The listing builds one solid part. Answer for the finished solid, in the listing's coordinates (mm). Face numbers are marked on the shaded views. Round coordinates to 2 decimals unless told otherwise and drop trailing zeros. Use a Markdown table: item, result. Add a question column.
Q1. Consider line 1 (Y direction, x = 0, z = 1.75) (1 decimal); line 2 (X direction, y = 39, z = 5.25); line 3 (Y direction, x = 20, z = 0.5). Determine where each line is inside the solid, lowest interval first.
Q2. Given pin 1 Ø5 at (y, z) = (62, 7.5) entering from +X; pin 2 Ø5 at (x, y) = (0, 133.35) entering from +Z; pin 3 Ø15 at (x, y) = (0.5, 5.5) entering from +Z, each flat-ended and moving along its own axis, determine where each tip first touches the part or whether it passes through.
Q3. For a pull along Z with two mould halves and no side action, classify the marked faces 1 and 2 as released by +Z, released by -Z, zero draft, split by the parting line, or undercut.
Q4. Section A-A on x = 48 is taken. Give the number of separate pieces and of enclosed holes in the cut face, then the cut area to 3 significant figures.
from build123d import *

# Parameters (mm, degrees)
SKETCH1_R           = 1.5875
BOSS_EXTRUDE1_DEPTH = 6.35
BOSS_EXTRUDE2_DEPTH = 133.35
CUT_EXTRUDE1_DEPTH  = 133.35
SKETCH5_RX          = 30.163516005
SKETCH5_RY          = 6.87067886
CUT_EXTRUDE2_DEPTH  = 216.619671093
BOSS_EXTRUDE3_DEPTH = 3.175
CUT_EXTRUDE3_START  = -7.9375
CUT_EXTRUDE3_DEPTH  = 7.9375
FILLET1_R           = 3.175


with BuildPart() as part:
    # Sketch1 → Boss-Extrude1 (new body)
    with BuildSketch(Plane.XY):
        with BuildLine():
            Line((150.084701559, -26.463982276), (6.230674922, -1.098636097))
            ThreePointArc((6.230674922, -1.098636097), (4.06678423, 4.846604717), (-2.163890692, 5.945240813))
            Line((-2.163890692, 5.945240813), (-52.123869843, 143.209155408))
            ThreePointArc((-52.123869843, 143.209155408), (97.960831716, 116.745173131), (150.084701559, -26.463982276))
        make_face()
        with Locations((0, 133.35)):
            Circle(SKETCH1_R, mode=Mode.SUBTRACT)
        with Locations((0, 107.95)):
            Circle(SKETCH1_R, mode=Mode.SUBTRACT)
        with Locations((85.715727752, 102.15202649)):
            Circle(SKETCH1_R, mode=Mode.SUBTRACT)
        with Locations((69.388922466, 82.694497635)):
            Circle(SKETCH1_R, mode=Mode.SUBTRACT)
        with Locations((131.324113864, 23.155984492)):
            Circle(SKETCH1_R, mode=Mode.SUBTRACT)
        with Locations((106.309996938, 18.745320779)):
            Circle(SKETCH1_R, mode=Mode.SUBTRACT)
        with Locations((0, 25.4)):
            Circle(SKETCH1_R, mode=Mode.SUBTRACT)
        with Locations((12.7, 21.997045256)):
            Circle(SKETCH1_R, mode=Mode.SUBTRACT)
        with Locations((21.997045256, 12.7)):
            Circle(SKETCH1_R, mode=Mode.SUBTRACT)
        with Locations((25.4, 0)):
            Circle(SKETCH1_R, mode=Mode.SUBTRACT)
    extrude(amount=BOSS_EXTRUDE1_DEPTH)

    # Sketch2 → Boss-Extrude2 (add)
    with BuildSketch(Plane(origin=(-52.123869843, 143.209155408, 0), x_dir=(0, 0, -1), z_dir=(-0.342020143325673, 0.939692620785907, 0))):
        with BuildLine():
            ThreePointArc((-4.7625, 0), (-3.175, 1.5875), (-1.5875, 0))
            Line((-1.5875, 0), (-4.7625, 0))
        make_face()
    extrude(amount=-BOSS_EXTRUDE2_DEPTH)

    # Sketch3 → Cut-Extrude1 (cut)
    with BuildSketch(Plane(origin=(150.084701559, -26.463982276, 0), x_dir=(0, 0, -1), z_dir=(-0.9848077530122086, 0.1736481776669274, 0))):
        with BuildLine():
            Line((-4.7625, 0), (-1.5875, 0))
            ThreePointArc((-1.5875, 0), (-3.175, -1.5875), (-4.7625, 0))
        make_face()
    extrude(amount=CUT_EXTRUDE1_DEPTH, mode=Mode.SUBTRACT)

    # Sketch5 → Cut-Extrude2 (cut, through all)
    with BuildSketch(Plane.XY.offset(6.35)):
        with Locations(Location((46.404952904, 127.496560255), (0, 0, 160))):
            Ellipse(SKETCH5_RX, SKETCH5_RY)
        with Locations(Location((117.501465515, 67.839502745), (0, 0, -60))):
            Ellipse(SKETCH5_RX, SKETCH5_RY)
        with Locations(Location((133.617736528, -23.560412051), (0, 0, -100))):
            Ellipse(SKETCH5_RX, SKETCH5_RY)
        with Locations(Location((87.212783624, -103.936148204), (0, 0, -140))):
            Ellipse(SKETCH5_RX, SKETCH5_RY)
        with Locations(Location((0, -135.679005491), (0, 0, 180))):
            Ellipse(SKETCH5_RX, SKETCH5_RY)
        with Locations(Location((-87.212783624, -103.936148204), (0, 0, 140))):
            Ellipse(SKETCH5_RX, SKETCH5_RY)
        with Locations(Location((-133.617736528, -23.560412051), (0, 0, 100))):
            Ellipse(SKETCH5_RX, SKETCH5_RY)
        with Locations(Location((-117.501465515, 67.839502746), (0, 0, 60))):
            Ellipse(SKETCH5_RX, SKETCH5_RY)
        with Locations(Location((-46.404952904, 127.496560255), (0, 0, 20))):
            Ellipse(SKETCH5_RX, SKETCH5_RY)
        with BuildLine():
            Line((57.978416111, 105.49005345), (23.39365582, 118.077876756))
            ThreePointArc((23.39365582, 118.077876756), (11.765579258, 116.547011434), (6.35, 106.143780472))
            Line((6.35, 106.143780472), (6.35, 34.892963227))
            ThreePointArc((6.35, 34.892963227), (10.52817209, 28.925915085), (17.564382214, 30.811261906))
            Line((17.564382214, 30.811261906), (63.363524719, 85.392554523))
            ThreePointArc((63.363524719, 85.392554523), (65.902018285, 96.842959039), (57.978416111, 105.49005345))
        make_face()
        with BuildLine():
            Line((112.221742786, 43.542261744), (93.819576202, 75.415749237))
            ThreePointArc((93.819576202, 75.415749237), (83.927931507, 81.717421903), (73.092289146, 77.22915188))
            Line((73.092289146, 77.22915188), (27.293146641, 22.647859263))
            ThreePointArc((27.293146641, 22.647859263), (26.658267541, 15.391157941), (33.260194783, 12.312628709))
            Line((33.260194783, 12.312628709), (103.428552014, 24.685203281))
            ThreePointArc((103.428552014, 24.685203281), (112.733329053, 31.82500982), (112.221742786, 43.542261744))
        make_face()
        with BuildLine():
            Line((113.955268805, -38.77943815), (120.34627419, -2.534245502))
            ThreePointArc((120.34627419, -2.534245502), (116.819471848, 8.651342476), (105.633883871, 12.178144818))
            Line((105.633883871, 12.178144818), (35.46552664, -0.194429754))
            ThreePointArc((35.46552664, -0.194429754), (30.314663336, -5.345293057), (33.393192568, -11.9472203))
            Line((33.393192568, -11.9472203), (95.098210342, -47.572628922))
            ThreePointArc((95.098210342, -47.572628922), (106.815462266, -48.084215189), (113.955268805, -38.77943815))
        make_face()
        with BuildLine():
            Line((62.367858079, -102.955807949), (90.561612985, -79.298438606))
            ThreePointArc((90.561612985, -79.298438606), (95.049883008, -68.462796245), (88.748210342, -58.57115155))
            Line((88.748210342, -58.57115155), (27.043192568, -22.945742928))
            ThreePointArc((27.043192568, -22.945742928), (19.786491246, -23.580622028), (17.901144426, -30.616832152))
            Line((17.901144426, -30.616832152), (42.270359152, -97.570699341))
            ThreePointArc((42.270359152, -97.570699341), (50.917453563, -105.494301515), (62.367858079, -102.955807949))
        make_face()
        with BuildLine():
            Line((-18.402166584, -118.958010982), (18.402166584, -118.958010982))
            ThreePointArc((18.402166584, -118.958010982), (28.805397546, -113.542431724), (30.336262868, -101.914355162))
            Line((30.336262868, -101.914355162), (5.967048142, -34.960487972))
            ThreePointArc((5.967048142, -34.960487972), (0, -30.782315882), (-5.967048142, -34.960487972))
            Line((-5.967048142, -34.960487972), (-30.336262868, -101.914355162))
            ThreePointArc((-30.336262868, -101.914355162), (-28.805397547, -113.542431723), (-18.402166584, -118.958010982))
        make_face()
        with BuildLine():
            Line((-90.561612985, -79.298438605), (-62.367858079, -102.955807949))
            ThreePointArc((-62.367858079, -102.955807949), (-50.917453563, -105.494301515), (-42.270359152, -97.570699341))
            Line((-42.270359152, -97.570699341), (-17.901144426, -30.616832152))
            ThreePointArc((-17.901144426, -30.616832152), (-19.786491246, -23.580622028), (-27.043192568, -22.945742928))
            Line((-27.043192568, -22.945742928), (-88.748210342, -58.57115155))
            ThreePointArc((-88.748210342, -58.57115155), (-95.049883008, -68.462796245), (-90.561612985, -79.298438605))
        make_face()
        with BuildLine():
            Line((-120.34627419, -2.534245501), (-113.955268805, -38.77943815))
            ThreePointArc((-113.955268805, -38.77943815), (-106.815462266, -48.084215189), (-95.098210342, -47.572628922))
            Line((-95.098210342, -47.572628922), (-33.393192568, -11.947220299))
            ThreePointArc((-33.393192568, -11.947220299), (-30.314663336, -5.345293057), (-35.46552664, -0.194429754))
            Line((-35.46552664, -0.194429754), (-105.633883871, 12.178144818))
            ThreePointArc((-105.633883871, 12.178144818), (-116.819471848, 8.651342476), (-120.34627419, -2.534245501))
        make_face()
        with BuildLine():
            Line((-93.819576202, 75.415749238), (-112.221742786, 43.542261745))
            ThreePointArc((-112.221742786, 43.542261745), (-112.733329053, 31.825009821), (-103.428552014, 24.685203281))
            Line((-103.428552014, 24.685203281), (-33.260194783, 12.312628709))
            ThreePointArc((-33.260194783, 12.312628709), (-26.658267541, 15.391157941), (-27.293146641, 22.647859263))
            Line((-27.293146641, 22.647859263), (-73.092289146, 77.229151881))
            ThreePointArc((-73.092289146, 77.229151881), (-83.927931506, 81.717421903), (-93.819576202, 75.415749238))
        make_face()
        with BuildLine():
            Line((-23.39365582, 118.077876756), (-57.978416111, 105.490053451))
            ThreePointArc((-57.978416111, 105.490053451), (-65.902018285, 96.842959039), (-63.363524718, 85.392554524))
            Line((-63.363524718, 85.392554524), (-17.564382214, 30.811261906))
            ThreePointArc((-17.564382214, 30.811261906), (-10.52817209, 28.925915085), (-6.35, 34.892963227))
            Line((-6.35, 34.892963227), (-6.35, 106.143780472))
            ThreePointArc((-6.35, 106.143780472), (-11.765579258, 116.547011434), (-23.39365582, 118.077876756))
        make_face()
    extrude(amount=-CUT_EXTRUDE2_DEPTH, mode=Mode.SUBTRACT)

    # Sketch6 → Boss-Extrude3 (add)
    with BuildSketch(Plane.XY.offset(6.35)):
        with BuildLine():
            Line((6.230674922, -1.098636097), (18.760587695, -3.307997785))
            ThreePointArc((18.760587695, -3.307997785), (12.245103965, 14.593146641), (-6.51548373, 17.901144426))
            Line((-6.51548373, 17.901144426), (-2.163890692, 5.945240813))
            ThreePointArc((-2.163890692, 5.945240813), (4.06678423, 4.846604717), (6.230674922, -1.098636097))
        make_face()
    extrude(amount=BOSS_EXTRUDE3_DEPTH)

    # Sketch7 → Cut-Extrude3 (cut)
    with BuildSketch(Plane.XY.offset(9.525).offset(CUT_EXTRUDE3_START)):
        with BuildLine():
            Line((6.230674922, -1.098636097), (15.633823079, -2.75666482))
            ThreePointArc((15.633823079, -2.75666482), (10.204253304, 12.160955535), (-5.429569775, 14.917620355))
            Line((-5.429569775, 14.917620355), (-2.163890692, 5.945240813))
            ThreePointArc((-2.163890692, 5.945240813), (4.06678423, 4.846604717), (6.230674922, -1.098636097))
        make_face()
    extrude(amount=CUT_EXTRUDE3_DEPTH, mode=Mode.SUBTRACT)

    # Fillet1
    fillet1_edges = [part.edges().sort_by_distance(p)[0] for p in [
        (12.245103965, 14.593146641, 6.35),
    ]]
    fillet(fillet1_edges, radius=FILLET1_R - 0.0001)  # a hair under: the kernel refuses the full size


solid = part.part
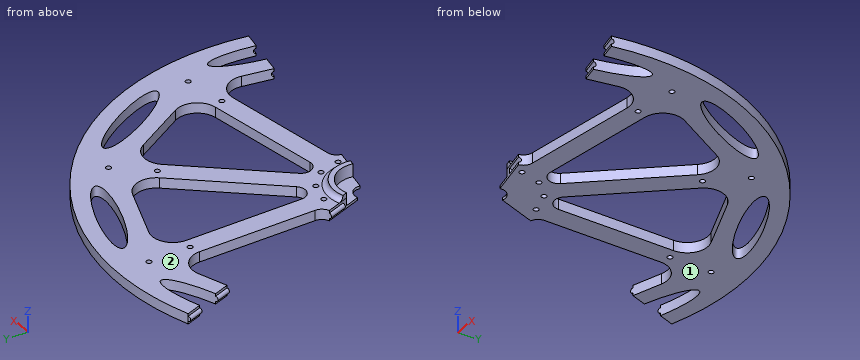
Checked values:
| question | item | result |
|---|---|---|
| 1 | line 1 | y = 15.9 to 23.8, 27 to 106.4, 109.5 to 131.8, 134.9 to 152.4 |
| 1 | line 2 | x = -6.35 to 6.35, 24.44 to 41.01, 113.79 to 147.33 |
| 1 | line 3 | y = -3.53 to 33.71, 118.81 to 133.84, 139.25 to 151.08 |
| 2 | pin 1 | stops at x = 140.19 |
| 2 | pin 2 | stops at z = 6.35 |
| 2 | pin 3 | stops at z = 1.59 |
| 3 | face 1 | released by -Z |
| 3 | face 2 | released by +Z |
| 4 | separate pieces | 4 |
| 4 | enclosed holes | 0 |
| 4 | area | 341 mm2 |
